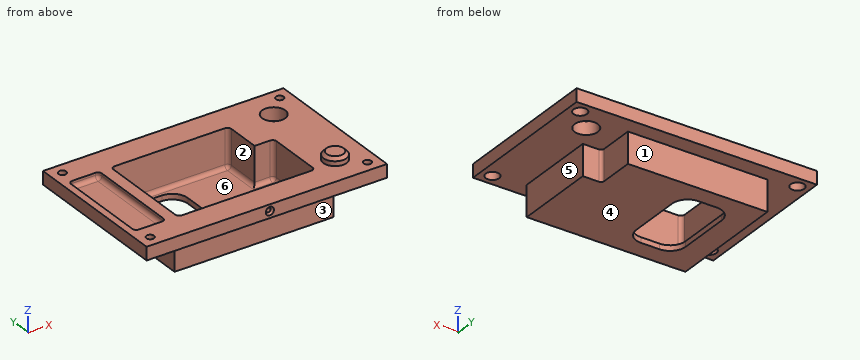
from build123d import *

# Parameters (mm, degrees)
F0_W            = 396.24
F0_H            = 248.92
F1_DEPTH        = 21.59
F3_DEPTH        = 50.8
F5_DEPTH        = 63.5
F6_R            = 6.35
F7_R            = 5.08
F8_W            = 81.28
F8_H            = 137.16
F9_DEPTH        = 72.391
F10_W           = 50.8
F10_H           = 160.02
F11_DEPTH       = 10.414
F12_R           = 6.35
F13_R           = 19.05
F14_DEPTH       = 12.7
F15_SIZE        = 5.08
F17_D           = 7.1374
F17_DEPTH       = 127
F17_CSINK_D     = 13.4874
F17_CSINK_ANGLE = 82
F17_TIP         = 2.1442912911
F19_D           = 12.7
F19_CBORE_D     = 22.225
F19_CBORE_DEPTH = 12.7
F20_R           = 19.05
F21_DEPTH       = 72.391
F22_R           = 25.4


with BuildPart() as f1:
    # F0 (on Top) → F1 (new body)
    with BuildSketch(Plane.XY):
        Rectangle(F0_W, F0_H)
    extrude(amount=-F1_DEPTH)

    # F2 (on face) → F3 (join)
    with BuildSketch(Plane(origin=(0, 0, -21.59), x_dir=(1, 0, 0), z_dir=(0, 0, -1))):
        Polygon((127, 99.06), (-134.62, 99.06), (-134.62, -97.79), (95.25, -97.79), (95.25, -35.56), (127, -35.56), align=None)
    extrude(amount=F3_DEPTH)

    # F4 (on face) → F5 (cut)
    with BuildSketch(Plane.XY):
        Polygon((-116.84, -81.28), (109.22, -81.28), (109.22, 17.78), (77.47, 17.78), (77.47, 80.01), (-116.84, 80.01), align=None)
    extrude(amount=-F5_DEPTH, mode=Mode.SUBTRACT)

    # F6
    f6_edges = [f1.edges().sort_by_distance(p)[0] for p in [
        (-3.81, -81.28, -63.5),
        (109.22, -31.75, -63.5),
        (93.345, 17.78, -63.5),
        (77.47, 48.895, -63.5),
        (-19.685, 80.01, -63.5),
        (-116.84, -0.635, -63.5),
        (109.22, -81.28, -31.75),
        (-116.84, -81.28, -31.75),
        (-116.84, 80.01, -31.75),
        (109.22, 17.78, -31.75),
        (77.47, 80.01, -31.75),
    ]]
    fillet(f6_edges, radius=F6_R)

    # F7
    f7_edges = [f1.edges().sort_by_distance(p)[0] for p in [
        (95.25, 35.56, -46.99),
    ]]
    fillet(f7_edges, radius=F7_R)

    # F8 (on face) → F9 (cut, through all)
    with BuildSketch(Plane(origin=(0, 0, -72.39), x_dir=(1, 0, 0), z_dir=(0, 0, -1))):
        with Locations((-55.88, 0)):
            Rectangle(F8_W, F8_H)
    extrude(amount=-F9_DEPTH, mode=Mode.SUBTRACT)

    # F10 (on face) → F11 (cut)
    with BuildSketch(Plane.XY):
        with Locations((-161.29, 0)):
            Rectangle(F10_W, F10_H)
    extrude(amount=-F11_DEPTH, mode=Mode.SUBTRACT)

    # F12
    f12_edges = [f1.edges().sort_by_distance(p)[0] for p in [
        (-135.89, 0, -10.414),
        (-161.29, 80.01, -10.414),
        (-186.69, 0, -10.414),
        (-161.29, -80.01, -10.414),
        (-186.69, 80.01, -5.207),
        (-135.89, 80.01, -5.207),
        (-135.89, -80.01, -5.207),
        (-186.69, -80.01, -5.207),
    ]]
    fillet(f12_edges, radius=F12_R)

    # F13 (on face) → F14 (join)
    with BuildSketch(Plane.XY):
        with Locations((147.32, -73.66)):
            Circle(F13_R)
    extrude(amount=F14_DEPTH)

    # F15
    f15_edges = [f1.edges().sort_by_distance(p)[0] for p in [
        (128.27, -73.66, 12.7),
    ]]
    chamfer(f15_edges, length=F15_SIZE)

    # F17
    with Locations(Plane.XZ.offset(124.46)):
        with Locations((5.08, -10.668)):
            CounterSinkHole(F17_D / 2, F17_CSINK_D / 2, depth=F17_DEPTH, counter_sink_angle=F17_CSINK_ANGLE)
            with Locations((0, 0, -(F17_DEPTH + F17_TIP / 2))):  # 118° drill point
                Cone(0, F17_D / 2, F17_TIP, mode=Mode.SUBTRACT)

    # F19 (through all)
    with Locations(Plane(origin=(0, 0, -21.59), x_dir=(1, 0, 0), z_dir=(0, 0, -1))):
        with Locations((-179.07, 105.41), (179.07, 105.41), (179.07, -105.41), (-179.07, -105.41)):
            CounterBoreHole(F19_D / 2, F19_CBORE_D / 2, F19_CBORE_DEPTH)

    # F20 (on face) → F21 (cut, through all)
    with BuildSketch(Plane.XY):
        with Locations((147.32, 73.66)):
            Circle(F20_R)
    extrude(amount=-F21_DEPTH, mode=Mode.SUBTRACT)

    # F22
    f22_edges = [f1.edges().sort_by_distance(p)[0] for p in [
        (-15.24, -68.58, -67.945),
        (-15.24, 68.58, -67.945),
        (-96.52, 68.58, -67.945),
        (-96.52, -68.58, -67.945),
    ]]
    fillet(f22_edges, radius=F22_R)


solid = f1.part
Check sheet for the modelled part. Datum: model origin and axes. Units: mm. Face numbers are marked on the shaded views. A direction names the side the tool comes from. Round coordinates to 2 decimals unless told otherwise and drop trailing zeros. Order: outer loops, then holes, each group sorted by start corner. A loop starts at its lowest first (then second) coordinate and runs counter-clockwise, first axis right, second up.
(1) Cross-section at C-C, the plane y = -34. Enter the section's corners in (x, z), and give its area (3 significant figures).
(2) Cross-section at B-B, the plane x = 147.32. Enter the section's corners in (y, z).
(3) Scan lines: probe 1 along Y at (x, z) = (179.07, -16); probe 2 along X at (y, z) = (-105.41, -3.75); probe 3 along Z at (x, y) = (5, -110). Record each from-to range of solid material in increasing order.
(4) Cross-section at A-A, the plane y = 105.41. Enter the section's corners in (x, z), and give its area (3 significant figures).
(5) Cross-section at D-D, the plane z = -48.5. Enter the section's corners in (x, y).
(6) Go/stop test with flat-tipped pins: P1, Ø12, axis at y = -76.5, z = -33.5, coming from the -X side; P2, Ø4.5, axis at x = -55, z = -69.5, coming from the +Y side; P3, Ø17, axis at x = -4.5, z = -37.5, coming from the -Y side; P4, Ø11.5, axis at x = 179.07, y = -105.41, coming from the +Z side. Record where each tip stops, or that it passes through.
(7) Draft check along X on the marked faces 4, 5 and 6. Enter one of: pulls with the +X half, pulls with the -X half, needs draft (parallel to the pull), parting line crosses it, or undercut.
(8) Access from +Z, -Z, +X, -X, +Y, -Y to the whole of each face (thin tool, end or side, straight path). Record for the marked faces 1, 2 and 3.
Check sheet entries:
1. outline: (-198.12, -21.59) - (-134.62, -21.59) - (-134.62, -72.39) - (-96.52, -72.39) - (-96.52, -63.5) - (-110.49, -63.5) arc R6.35 cw to (-116.84, -57.15) - (-116.84, 0) - (-135.89, 0) - (-135.89, -4.06) arc R6.35 cw to (-142.24, -10.41) - (-180.34, -10.41) arc R6.35 cw to (-186.69, -4.06) - (-186.69, 0) - (-198.12, 0) - close; (-15.24, -72.39) - (127, -72.39) - (127, -21.59) - (198.12, -21.59) - (198.12, 0) - (109.22, 0) - (109.22, -57.15) arc R6.35 cw to (102.87, -63.5) - (-15.24, -63.5) - close
1. area: 6,270 mm2
2. outline: (-124.46, -21.59) - (54.61, -21.59) - (54.61, 0) - (-54.61, 0) - (-54.61, 7.62) - (-59.69, 12.7) - (-87.63, 12.7) - (-92.71, 7.62) - (-92.71, 0) - (-124.46, 0) - close; (92.71, -21.59) - (124.46, -21.59) - (124.46, 0) - (92.71, 0) - close
3. probe 1: y = -124.46 to -116.52, -94.3 to 94.3, 116.52 to 124.46
3. probe 2: x = -198.12 to -185.42, -172.72 to 172.72, 185.42 to 198.12
3. probe 3: z = -21.59 to -14.24, -7.1 to 0
4. outline: (-198.12, -21.59) - (-190.18, -21.59) - (-190.18, -8.89) - (-185.42, -8.89) - (-185.42, 0) - (-198.12, 0) - close; (-172.72, -8.89) - (-167.96, -8.89) - (-167.96, -21.59) - (167.96, -21.59) - (167.96, -8.89) - (172.72, -8.89) - (172.72, 0) - (-172.72, 0) - close; (185.42, -8.89) - (190.18, -8.89) - (190.18, -21.59) - (198.12, -21.59) - (198.12, 0) - (185.42, 0) - close
4. area: 7,760 mm2
5. outline: (-134.62, -99.06) - (127, -99.06) - (127, 35.56) - (100.33, 35.56) arc R5.08 cw to (95.25, 40.64) - (95.25, 97.79) - (-134.62, 97.79) - close; hole (-116.84, -74.93) arc R6.35 ccw to (-110.49, -81.28) - (102.87, -81.28) arc R6.35 ccw to (109.22, -74.93) - (109.22, 11.43) arc R6.35 ccw to (102.87, 17.78) - (77.47, 17.78) - (77.47, 73.66) arc R6.35 ccw to (71.12, 80.01) - (-110.49, 80.01) arc R6.35 ccw to (-116.84, 73.66) - close
6. P1: stops at x = -134.62
6. P2: stops at y = 97.79
6. P3: stops at y = -99.06
6. P4: passes through
7. face 4: needs draft
7. face 5: pulls with the +X half
7. face 6: undercut
8. face 1: -Z, +X, -X, +Y
8. face 2: +Z
8. face 3: -Z, +X, -X, -Y
